Geometry check sheet. Reference: drawing and pictorial views, mm from the part's lowest x, y, z. Round coordinates to 2 decimals unless told otherwise and drop trailing zeros. Write each loop counter-clockwise with the first axis right and the second up, starting at its lowest first coordinate (ties: lowest second). Pieces come first, ordered by that corner, then holes. Notation, with made-up numbers: (-32, -39.75) -> (11, -39.75) arc R33 cw to (11, -6.75) -> close; hole circle Ø5 at (27, 71). An arc over 180 degrees is marked (long way). Write item = value, one per line.
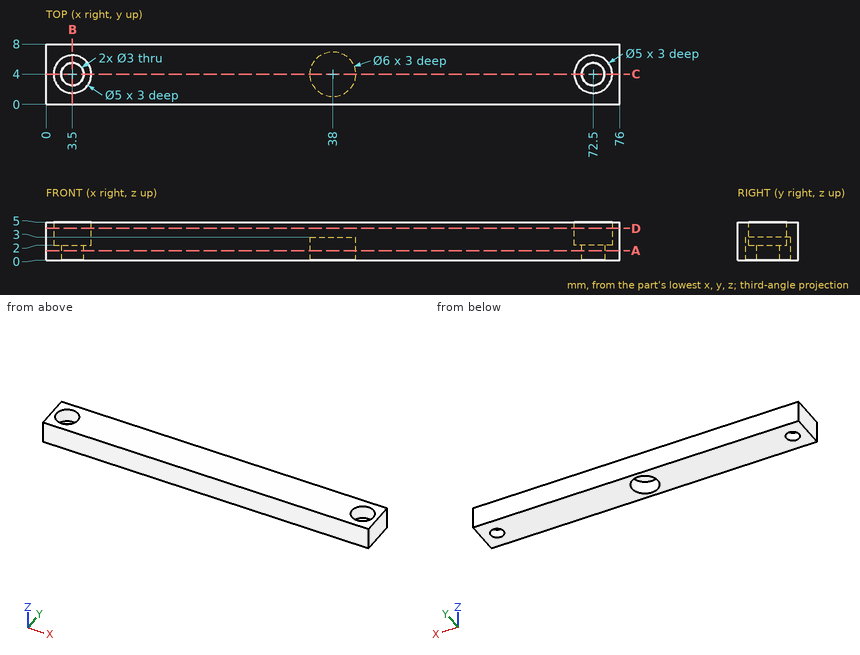
(1) Sectioned sample at D-D on z = 4.2. Enter the section's corners in (x, y), then the cut area to 3 significant figures.
Worked answers:
outline = (0, 0) -> (76, 0) -> (76, 8) -> (0, 8) -> close; hole circle Ø5 at (3.5, 4); hole circle Ø5 at (72.5, 4)
area = 569 mm²
(2) Sectioned sample at B-B on x = 3.5. Enter the section's corners in (y, z).
Worked answers:
outline = (0, 0) -> (2.5, 0) -> (2.5, 2) -> (1.5, 2) -> (1.5, 5) -> (0, 5) -> close; (5.5, 0) -> (8, 0) -> (8, 5) -> (6.5, 5) -> (6.5, 2) -> (5.5, 2) -> close
(3) Go/stop test with a flat-tipped pin: P1, Ø2.5, axis at x = 3, y = 3.5, coming from the +Z side. Record where the tip stops, or that it passes through.
Worked answers:
P1 = 2
(4) Sectioned sample at C-C on y = 4. Enter the section's corners in (x, z).
Worked answers:
outline = (0, 0) -> (2, 0) -> (2, 2) -> (1, 2) -> (1, 5) -> (0, 5) -> close; (5, 0) -> (35, 0) -> (35, 3) -> (41, 3) -> (41, 0) -> (71, 0) -> (71, 2) -> (70, 2) -> (70, 5) -> (6, 5) -> (6, 2) -> (5, 2) -> close; (74, 0) -> (76, 0) -> (76, 5) -> (75, 5) -> (75, 2) -> (74, 2) -> close
(5) Sectioned sample at A-A on z = 1.25. Enter the section's corners in (x, y).
Worked answers:
outline = (0, 0) -> (76, 0) -> (76, 8) -> (0, 8) -> close; hole circle Ø3 at (3.5, 4); hole circle Ø6 at (38, 4); hole circle Ø3 at (72.5, 4)
(6) Material ranges on L1, parallel to Y at x = 38, z = 1.8; L2, parallel to X at y = 4.5, z = 3.7; L3, parallel to Y at x = 3.5, z = 3.55, recorded low to high. Write a range as [from, to].
Worked answers:
L1 = [0, 1], [7, 8]
L2 = [0, 1.05], [5.95, 70.05], [74.95, 76]
L3 = [0, 1.5], [6.5, 8]
